Design review of the part built by this model. Coordinates are the model's own, in mm. Face numbers are marked on the shaded views. A direction names the side the tool comes from. Give positions to 0.01 mm unless a question says otherwise; leave off trailing zeros. Write each loop counter-clockwise with the first axis right and the second up, starting at its lowest first coordinate (ties: lowest second). Pieces come first, ordered by that corner, then holes. Notation, with made-up numbers: M -33,34 L 8,34 A25 ccw 8,64 Z; hole C 69,56 d1. An arc over 180 degrees is marked long. Answer in a Markdown table with one row per item.
```python
from build123d import *

# Parameters (mm, degrees)
TAPPED_HOLE_FOR_10_32_HELICOIL1_D = 5.1054
CIRPATTERN1_COUNT                 = 4


with BuildPart() as part:
    # Sketch1 → Revolve1 (revolve)
    with BuildSketch(Plane.XY, mode=Mode.PRIVATE) as revolve1_sk:
        Polygon((31.8135, 0), (38.1, 0), (38.1, 52.07), (50.8, 52.07), (50.8, 58.42), (33.3883, 58.42), (33.3883, 57.15), (31.2801, 57.15), (31.2801, 58.42), (27.051, 58.42), (27.051, 33.02), (25.4, 33.02), (25.4, 31.75), (31.8135, 31.75), (31.8135, 28.702), (34.582975987, 28.702), (34.582975987, 25.146), (31.8135, 25.146), (31.8135, 6.096), (33.909, 6.096), (33.909, 2.54), (31.8135, 2.54), align=None)
    revolve(revolve1_sk.sketch.rotate(Axis((0, 0, 0), (0, 1, 0)), 90), axis=Axis((0, 0, 0), (0, 1, 0)))

    # Tapped Hole for #10-32 Helicoil1 (through all)
    with Locations(Plane(origin=(0, 58.42, 0), x_dir=(1, 0, 0), z_dir=(0, 1, 0))):
        with Locations((0, 44.45)):
            tapped_hole_for_10_32_helicoil1 = Hole(TAPPED_HOLE_FOR_10_32_HELICOIL1_D / 2)

    # CirPattern1: Tapped Hole for #10-32 Helicoil1 ×4 about axis
    cirpattern1_axis = Axis((0, 0, 0), (0, 1, 0))
    for i in range(1, CIRPATTERN1_COUNT):
        add(tapped_hole_for_10_32_helicoil1.rotate(cirpattern1_axis, i * 360 / CIRPATTERN1_COUNT), mode=Mode.SUBTRACT)


solid = part.part
```
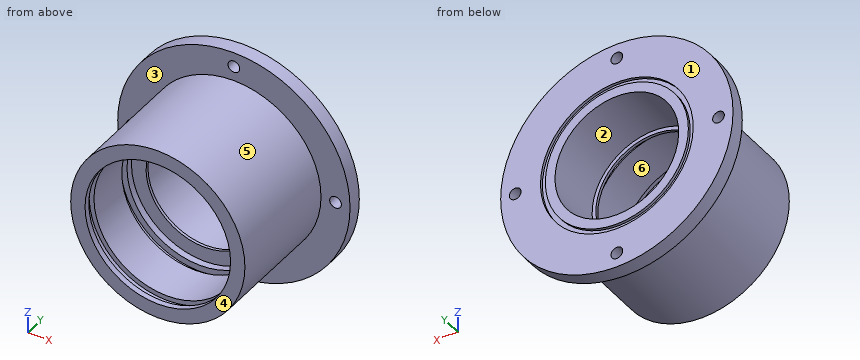
1) Add section C-C (y = 40). Write out the cut boundary in (x, z), and give its area (3 significant figures).
Geometry says:
| item | result |
|---|---|
| outline | C 0,0 d76.2; hole C 0,0 d54.1 |
| area | 2,260 mm^2 |
2) Add section D-D (z = 0). Count the separate pieces of the cut face and the enclosed holes in it, and give its area (3 significant figures).
Geometry says:
| item | result |
|---|---|
| separate pieces | 4 |
| enclosed holes | 0 |
| area | 1,050 mm^2 |
3) For the marked faces 1, 2 and 3, list the 3-axis set-ups (+Z, -Z, +X, -X, +Y, -Y) from which the entire face can be reached by the end or side of a thin tool; tool diameter is ignored.
Geometry says:
| item | result |
|---|---|
| face 1 | +Z, -Z, +X, -X, +Y |
| face 2 | +Y |
| face 3 | -Y |
4) The part is to be moulded in two halves that separate along Z. For the marked faces 4, 5 and 6, say which applies: released by +Z, released by -Z, zero draft, split by the parting line, or undercut.
Geometry says:
| item | result |
|---|---|
| face 4 | zero draft |
| face 5 | split by the parting line |
| face 6 | undercut |
5) Insertion check: P1, Ø1.5, axis at x = 21, y = 9, coming from the -Z side; P2, Ø10, axis at y = 50, z = -21.5, coming from the -X side; P3, Ø10, axis at x = -39.5, y = 40.5, coming from the -Z side; P4, Ø20.5, axis at x = -14.5, z = 3, coming from the +Y side. Each pin has a flat end and moves straight along its axis. Give the tip position at first contact, or say it passes through.
Geometry says:
| item | result |
|---|---|
| P1 | z = -32.27 |
| P2 | x = -47.89 |
| P3 | z = -16.17 |
| P4 | through |
6) Add section B-B (z = 44.45). Write out the cut boundary in (x, y), and give its area (3 significant figures).
Geometry says:
| item | result |
|---|---|
| outline | M -24.59,52.07 L -2.55,52.07 L -2.55,58.42 L -24.59,58.42 Z; M 2.55,52.07 L 24.59,52.07 L 24.59,58.42 L 2.55,58.42 Z |
| area | 280 mm^2 |
7) Add section A-A (x = -44.45). Write out the cut boundary in (y, z), and give its area (3 significant figures).
Geometry says:
| item | result |
|---|---|
| outline | M 52.07,-24.59 L 58.42,-24.59 L 58.42,-2.55 L 52.07,-2.55 Z; M 52.07,2.55 L 58.42,2.55 L 58.42,24.59 L 52.07,24.59 Z |
| area | 280 mm^2 |
8) To check wall thickness, follow probe 1 along X at (y, z) = (57.65, 0); probe 2 along X at (y, z) = (55.5, 0); probe 3 along Z at (x, y) = (4, 19.5). State the ranges of each line that lie inside material, in increasing order. Write a range as [from, to].
Geometry says:
| item | result |
|---|---|
| probe 1 | [-50.8, -47], [-41.9, -33.39], [-31.28, -27.05], [27.05, 31.28], [33.39, 41.9], [47, 50.8] |
| probe 2 | [-50.8, -47], [-41.9, -27.05], [27.05, 41.9], [47, 50.8] |
| probe 3 | [-37.89, -31.56], [31.56, 37.89] |
